Source: CAD feature listing. Evaluate the final solid. Frame: model axes, mm. Face numbers are marked on the shaded views. A direction names the side the tool comes from. Give positions to 0.01 mm unless a question says otherwise; leave off trailing zeros. Loops run counter-clockwise (first coordinate to the right, second up) from the corner with the lowest first, then second, coordinate; pieces in that order, holes last. Notation, with made-up numbers: M -38,23 L 19,23 A33 cw 19,58 Z; hole C 83,3 d4. An arc over 180 degrees is marked long. Put each result on its own line as item: value. Start each with the question number.
```python
from build123d import *

# Parameters (mm, degrees)
SKETCH_1_R          = 1.5
EXTRUDE_1_DEPTH     = 2.8
EXTRUDE_2_DEPTH     = 15.5
SKETCH_3_W          = 24
SKETCH_3_H          = 50
EXTRUDE_3_DEPTH     = 4.2
SKETCH_4_R          = 16
CUT_EXTRUDE_4_DEPTH = 30
FILLET_1_R          = 3


with BuildPart() as part:
    # Эскиз1 → Вытянуть1 (new body)
    with BuildSketch(Plane(origin=(0, 0, 0), x_dir=(1, 0, 0), z_dir=(0, 1, 0))):
        with BuildLine():
            Line((0, 22), (0, 17))
            Line((0, 17), (-26, 17))
            Line((-26, 17), (-26, 0))
            Line((-26, 0), (-26, -17))
            Line((-26, -17), (0, -17))
            Line((0, -17), (0, -22))
            ThreePointArc((0, -22), (1.94635486, -25.432570704), (5.891270819, -25.524641072))
            Line((5.891270819, -25.524641072), (46.891270819, -3.524641072))
            ThreePointArc((46.891270819, -3.524641072), (49, 0), (46.891270819, 3.524641072))
            Line((46.891270819, 3.524641072), (5.891270819, 25.524641072))
            ThreePointArc((5.891270819, 25.524641072), (1.94635486, 25.432570704), (0, 22))
        make_face()
        with Locations(Location((4, 22, 0), (0, 0, 270))):
            Circle(SKETCH_1_R, mode=Mode.SUBTRACT)
        with Locations(Location((4, -22, 0), (0, 0, 270))):
            Circle(SKETCH_1_R, mode=Mode.SUBTRACT)
        with Locations(Location((45, 0, 0), (0, 0, 270))):
            Circle(SKETCH_1_R, mode=Mode.SUBTRACT)
    extrude(amount=EXTRUDE_1_DEPTH)

    # Эскиз2 → Вытянуть2 (add)
    with BuildSketch(Plane(origin=(0, 2.8, 0), x_dir=(1, 0, 0), z_dir=(0, 1, 0))):
        Polygon((-2, 17.022348164), (-26, 17), (-26, -17), (-2, -17), align=None)
    extrude(amount=EXTRUDE_2_DEPTH)

    # Эскиз3 → Вытянуть3 (add)
    with BuildSketch(Plane(origin=(0, 18.3, 0), x_dir=(1, 0, 0), z_dir=(0, 1, 0))):
        with Locations((-14, 0.011174082)):
            Rectangle(SKETCH_3_W, SKETCH_3_H)
    extrude(amount=EXTRUDE_3_DEPTH)

    # Эскиз4 → Вытянуть4 (cut)
    with BuildSketch(Plane.ZY.offset(26)):
        with Locations((0, 18)):
            Circle(SKETCH_4_R)
    extrude(amount=-CUT_EXTRUDE_4_DEPTH, mode=Mode.SUBTRACT)

    # Скругление1
    fillet_1_edges = [part.edges().sort_by_distance(p)[0] for p in [
        (-14, 18.3, -17.011174082),
        (-14, 18.3, 17),
    ]]
    fillet(fillet_1_edges, radius=FILLET_1_R)


solid = part.part
```
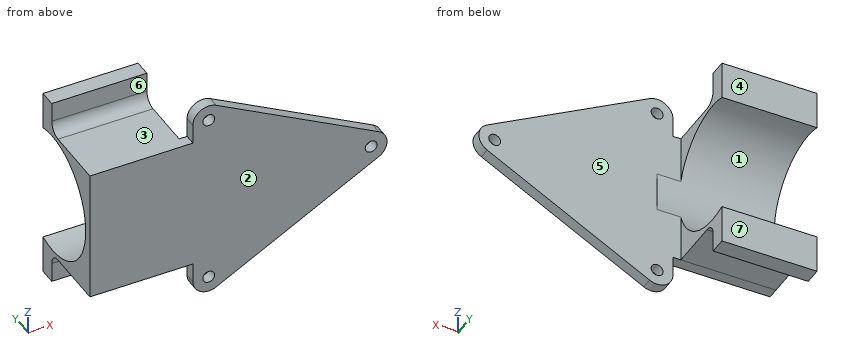
1. Section C-C, the plane x = 45. Output: boundary loops of the cut face in (y, z).
2. Section D-D, the plane z = -9.5. Output: boundary loops of the cut face in (x, y), plus the area to 3 significant figures.
3. Contact query for flat-ended pins moving along their axis: pin 1 (0.8 mm diameter, centred on y = 2, z = 18.5, fed in from -X); pin 2 (5 mm diameter, centred on x = 0.5, z = -2, fed in from +Y); pin 3 (4 mm diameter, centred on x = 4, z = -22, fed in from +Y); pin 4 (2.5 mm diameter, centred on x = 4, z = 22, fed in from -Y). Output: stop coordinate, or through.
4. Section B-B, the plane y = 9. Output: boundary loops of the cut face in (x, z).
5. Set-up query: the marked faces 5, 6 and 7. Return all of +Z, -Z, +X, -X, +Y, -Y with unobstructed straight access to the full face (end or side cutting, diameter ignored); none if empty.
6. Section A-A, the plane z = 0. Output: boundary loops of the cut face in (x, y).
7. Ray query, line 1 (Y direction, x = 1.5, z = -5); line 2 (Z direction, x = -18, y = 8.5); line 3 (Z direction, x = -14, y = 8). Return the intervals inside material, ascending.
8. Pull-direction query (Y, two-part tool) for the marked faces 1, 2, 3 and 4; classes: released by +Y, released by -Y, zero draft, split by the parting line, or undercut.
Results found:
1. outline: M 0,-4.54 L 2.8,-4.54 L 2.8,-1.5 L 0,-1.5 Z; M 0,1.5 L 2.8,1.5 L 2.8,4.54 L 0,4.54 Z
2. outline: M -26,0 L 35.76,0 L 35.76,2.8 L -2,2.8 L -2,5.13 L -26,5.13 Z
2. area: 229 mm²
3. pin 1: x = 0
3. pin 2: y = 2.65
3. pin 3: y = 2.8
3. pin 4: through
4. outline: M -26,-17 L -2,-17.02 L -2,-13.23 L -26,-13.23 Z; M -26,13.23 L -2,13.23 L -2,17 L -26,17 Z
5. face 5: +Z, -Z, +X, +Y
5. face 6: +Z, +X, -X, -Y
5. face 7: +Z, -Z, +X, -X, +Y
6. outline: M -26,0 L 43.5,0 L 43.5,2.8 L 4,2.8 L 4,2 L -26,2 Z; M 46.5,0 L 49,0 L 49,2.8 L 46.5,2.8 Z
7. line 1: 0 to 2.8
7. line 2: -17.01 to -12.87, 12.87 to 17
7. line 3: -17.01 to -12.49, 12.49 to 17
8. face 1: undercut
8. face 2: released by -Y
8. face 3: zero draft
8. face 4: released by +Y
